Autodesk Fusion 360 part; units mm, degrees
sketch "Esquisse1" plane through (0, 0, 0) normal (0, 1, 0) x (1, 0, 0)
  circle A0 centre (0, 0) radius 20
  circle A1 centre (0, 0) radius 3.1
  line L0 (-2.1, -2.2804) -> (-2.1, 2.2804)
  line L1 (2.1, -2.2804) -> (2.1, 2.2804)
  line L2 (0, 0) -> (0, -3.1) construction
  line L3 (0, 0) -> (0, 3.1) construction
  dimension "d1" = 40
  dimension "d4" = 6.2
  dimension "d5" = 4.2
extrude "Extrusion1" add sketch "Esquisse1" along normal blind 7 contours A0 | A1 L1 | A1 L0
sketch "Esquisse2" plane through (0, 0, 0) normal (0, -1, 0) x (1, 0, 0)
  arc A0 (2.1, 2.2804) -> (-2.1, 2.2804) centre (0, 0) ccw
  line L0 (2.1, 2.2804) -> (2.1, -2.2804)
  arc A1 (-2.1, -2.2804) -> (2.1, -2.2804) centre (0, 0) ccw
  line L1 (-2.1, -2.2804) -> (-2.1, 2.2804)
  circle A2 centre (0, 0) radius 20
extrude "Extrusion2" add sketch "Esquisse2" against normal blind 4 contours A0 L0 A1 L1
hole "Perçage1" at (0, 0, 0) direction (0, 1, 0) diameter 2.4 depth 23 tip angle 118
sketch "Esquisse3" plane through (0, 7, 0) normal (0, 1, 0) x (-1, 0, 0)
  arc A0 (2.1, 2.2804) -> (-2.1, 2.2804) centre (0, 0) ccw
  line L0 (2.1, 2.2804) -> (2.1, -2.2804)
  arc A1 (-2.1, -2.2804) -> (2.1, -2.2804) centre (0, 0) ccw
  line L1 (-2.1, -2.2804) -> (-2.1, 2.2804)
  circle A2 centre (0, 0) radius 20
  arc A3 (2.1, 2.2804) -> (-2.1, 2.2804) centre (0, 0) ccw
  line L2 (-2.1, 2.2804) -> (-2.1, -2.2804)
  arc A4 (-2.1, -2.2804) -> (2.1, -2.2804) centre (0, 0) ccw
  line L3 (2.1, -2.2804) -> (2.1, 2.2804)
  arc A5 (-3.1, -2.6833) -> (3.1, -2.6833) centre (0, 0) ccw
  line L4 (3.1, 2.6833) -> (3.1, -2.6833)
  arc A6 (3.1, 2.6833) -> (-3.1, 2.6833) centre (0, 0) ccw
  line L5 (-3.1, -2.6833) -> (-3.1, 2.6833)
  circle A7 centre (0, 0) radius 1.2
  dimension "d11" = -1
extrude "Extrusion3" add sketch "Esquisse3" along normal blind 6 contours A5 L4 A6 L5
fillet "Congé1" radius 2 4 edges at (3.1, 10, 2.6833) (3.1, 10, -2.6833) (-3.1, 10, 2.6833) (-3.1, 10, -2.6833)
fillet "Congé2" radius 6 8 edges at (3.1, 7, 0) (2.8457, 7, 2.7648) (0, 7, 4.1) (-2.8457, 7, 2.7648) (-3.1, 7, 0) (-2.8457, 7, -2.7648) (0, 7, -4.1) (2.8457, 7, -2.7648)
sketch "Esquisse4" plane through (0, 7, 0) normal (0, 1, 0) x (-1, 0, 0)
  circle A0 centre (0, 0) radius 20
  line L0 (-9.1, -1.7889) -> (-9.1, 1.7889)
  arc A1 (-5.2905, 8.6035) -> (-9.1, 1.7889) centre (-1.1, 1.7889) ccw
  arc A2 (5.2905, 8.6035) -> (-5.2905, 8.6035) centre (0, 0) ccw
  arc A3 (9.1, 1.7889) -> (5.2905, 8.6035) centre (1.1, 1.7889) ccw
  line L1 (9.1, 1.7889) -> (9.1, -1.7889)
  arc A4 (5.2905, -8.6035) -> (9.1, -1.7889) centre (1.1, -1.7889) ccw
  arc A5 (-5.2905, -8.6035) -> (5.2905, -8.6035) centre (0, 0) ccw
  arc A6 (-9.1, -1.7889) -> (-5.2905, -8.6035) centre (-1.1, -1.7889) ccw
  circle A7 centre (0, 0) radius 20
  circle A8 centre (0, 0) radius 10.25
  line L2 (0, 0) -> (0, 20) construction
  line L3 (0, 10.25) -> (0, 20) construction
  circle A9 centre (0, 0) radius 18
  line L4 (2.5, 12) -> (2.5, 16)
  arc A10 (2.5, 16) -> (-2.5, 16) centre (0, 16) ccw
  line L5 (-2.5, 16) -> (-2.5, 12)
  arc A11 (-2.5, 12) -> (2.5, 12) centre (0, 12) ccw
  line L6 (0, 12) -> (0, 16) construction
  arc A12 (-1.5, 12) -> (1.5, 12) centre (0, 12) ccw
  line L7 (1.5, 12) -> (1.5, 16)
  arc A13 (1.5, 16) -> (-1.5, 16) centre (0, 16) ccw
  line L8 (-1.5, 16) -> (-1.5, 12)
  line L9 (-15.9894, 2.5666) -> (-12.1852, 1.3306)
  line L10 (-15.6804, 3.5177) -> (-11.8762, 2.2816)
  arc A14 (-14.7534, 6.3709) -> (-15.6804, 3.5177) centre (-15.2169, 4.9443) ccw
  arc A15 (-14.4444, 7.3219) -> (-15.9894, 2.5666) centre (-15.2169, 4.9443) ccw
  line L11 (-10.6401, 6.0858) -> (-14.4444, 7.3219)
  line L12 (-10.9492, 5.1348) -> (-14.7534, 6.3709)
  arc A16 (-11.8762, 2.2816) -> (-10.9492, 5.1348) centre (-11.4127, 3.7082) ccw
  arc A17 (-12.1852, 1.3306) -> (-10.6401, 6.0858) centre (-11.4127, 3.7082) ccw
  line L13 (-7.382, -14.4137) -> (-5.0309, -11.1777)
  line L14 (-8.191, -13.8259) -> (-5.8399, -10.5899)
  arc A18 (-10.6181, -12.0626) -> (-8.191, -13.8259) centre (-9.4046, -12.9443) ccw
  arc A19 (-11.4271, -11.4748) -> (-7.382, -14.4137) centre (-9.4046, -12.9443) ccw
  line L15 (-9.076, -8.2387) -> (-11.4271, -11.4748)
  line L16 (-8.2669, -8.8265) -> (-10.6181, -12.0626)
  arc A20 (-5.8399, -10.5899) -> (-8.2669, -8.8265) centre (-7.0534, -9.7082) ccw
  arc A21 (-5.0309, -11.1777) -> (-9.076, -8.2387) centre (-7.0534, -9.7082) ccw
  line L17 (11.4271, -11.4748) -> (9.076, -8.2387)
  line L18 (10.6181, -12.0626) -> (8.2669, -8.8265)
  arc A22 (8.191, -13.8259) -> (10.6181, -12.0626) centre (9.4046, -12.9443) ccw
  arc A23 (7.382, -14.4137) -> (11.4271, -11.4748) centre (9.4046, -12.9443) ccw
  line L19 (5.0309, -11.1777) -> (7.382, -14.4137)
  line L20 (5.8399, -10.5899) -> (8.191, -13.8259)
  arc A24 (8.2669, -8.8265) -> (5.8399, -10.5899) centre (7.0534, -9.7082) ccw
  arc A25 (9.076, -8.2387) -> (5.0309, -11.1777) centre (7.0534, -9.7082) ccw
  line L21 (14.4444, 7.3219) -> (10.6401, 6.0858)
  line L22 (14.7534, 6.3709) -> (10.9492, 5.1348)
  arc A26 (15.6804, 3.5177) -> (14.7534, 6.3709) centre (15.2169, 4.9443) ccw
  arc A27 (15.9894, 2.5666) -> (14.4444, 7.3219) centre (15.2169, 4.9443) ccw
  line L23 (12.1852, 1.3306) -> (15.9894, 2.5666)
  line L24 (11.8762, 2.2816) -> (15.6804, 3.5177)
  arc A28 (10.9492, 5.1348) -> (11.8762, 2.2816) centre (11.4127, 3.7082) ccw
  arc A29 (10.6401, 6.0858) -> (12.1852, 1.3306) centre (11.4127, 3.7082) ccw
  dimension "d18" = 20.5
  dimension "d19" = -2
  dimension "d20" = 16
  dimension "d21" = 12
  dimension "d22" = 5
  dimension "d23" = -1
  dimension "d25" = 360
extrude "Extrusion5" add 1 faces at (13.6578, 0, 1.0235) along direction (0, -1, 0) blind 3
extrude "Extrusion6" add 1 faces at (13.6578, -3, 1.0235) along direction (0, -1, 0) blind 5
extrude "Extrusion7" cut 1 faces at (-1.7989, 4, 0.0299) along direction (0, -1, 0) blind 10
fillet "Congé4" radius 2 2 edges at (-18.6465, -8, -7.2323) (-18.6465, 7, 7.2323)
Geometry check sheet. Reference: the model listing, model coordinates, mm. A direction names the side the tool comes from. Give positions to 0.01 mm unless a question says otherwise; leave off trailing zeros. Loops run counter-clockwise (first coordinate to the right, second up) from the corner with the lowest first, then second, coordinate; pieces in that order, holes last. Notation, with made-up numbers: (35.5, -29) -> (42.5, -29) arc R17 cw to (42.5, 3) -> close; hole circle Ø8 at (19.5, -16.75). An arc over 180 degrees is marked (long way). Answer in a Markdown table with one row per item. Add a question column.
1) Draft check along Z on faces 1 (the face through (-2.1, 4, 0)), 2 (the face through (8, 7, 8)), 3 (the face through (-4.336, -0.423, 19.524)). Enter one of: pulls with the +Z half, pulls with the -Z half, needs draft (parallel to the pull), parting line crosses it, or undercut.
2) Cross-section at C-C on y = -3.75. Record the boundary of the cut face in (x, z), and give its area (3 significant figures).
3) Set-up check for faces 4 (the face through (0, 10, -3.1)), 5 (the face through (-4.811, 8.804, -0.025)): record each of +Z, -Z, +X, -X, +Y, -Y from which the full face is reachable in a straight line by a thin tool's end or side.
4) Material ranges on probe 1 along Y at (x, z) = (-14, -8); probe 2 along X at (y, z) = (-6.95, 0); probe 3 along Z at (x, y) = (0, -7.5), recorded low to high. Write a range as from..to.
5) Cross-section at D-D on y = 8. Record the boundary of the cut face in (x, z), and give its area (3 significant figures).
6) Gauge pin test, flat ends, axial feed: P1, Ø8, axis at x = 1, y = -1, coming from the +Z side; P2, Ø1.4, axis at y = 6, z = -0.5, coming from the +X side; P3, Ø2, axis at y = -3.5, z = 11.5, coming from the -X side; P4, Ø11, axis at x = 1.5, z = 2, coming from the +Y side. Record the tip position at first contact, or that the pin passes through.
Outcome:
| question | item | result |
|---|---|---|
| 1 | face 1 | undercut |
| 1 | face 2 | needs draft |
| 1 | face 3 | parting line crosses it |
| 2 | outline | circle Ø40 at (0, 0); hole (-2.1, -2.28) arc R3.1 ccw to (2.1, -2.28) -> (2.1, 2.28) arc R3.1 ccw to (-2.1, 2.28) -> close |
| 2 | area | 1,230 mm^2 |
| 3 | face 4 | +Y |
| 3 | face 5 | +Z, -Z, -X, +Y |
| 4 | probe 1 | y = -8..7 |
| 4 | probe 2 | x = -19.76..-1.2, 1.2..19.76 |
| 4 | probe 3 | z = -19.32..-1.2, 1.2..19.32 |
| 5 | outline | (-5.78, -1.79) arc R4.68 ccw to (-3.55, -5.78) arc R6.78 ccw to (3.55, -5.78) arc R4.68 ccw to (5.78, -1.79) -> (5.78, 1.79) arc R4.68 ccw to (3.55, 5.78) arc R6.78 ccw to (-3.55, 5.78) arc R4.68 ccw to (-5.78, 1.79) -> close; hole (-2.1, -2.28) arc R3.1 ccw to (2.1, -2.28) -> (2.1, 2.28) arc R3.1 ccw to (-2.1, 2.28) -> close |
| 5 | area | 109 mm^2 |
| 6 | P1 | stops at z = 20 |
| 6 | P2 | stops at x = 19.97 |
| 6 | P3 | stops at x = -17.02 |
| 6 | P4 | stops at y = 13 |
